The listing builds one solid part. Answer for the finished solid, in the listing's coordinates (mm). Face numbers are marked on the shaded views. A direction names the side the tool comes from. Round coordinates to 2 decimals unless told otherwise and drop trailing zeros. Write each loop counter-clockwise with the first axis right and the second up, starting at its lowest first coordinate (ties: lowest second). Pieces come first, ordered by that corner, then holes.
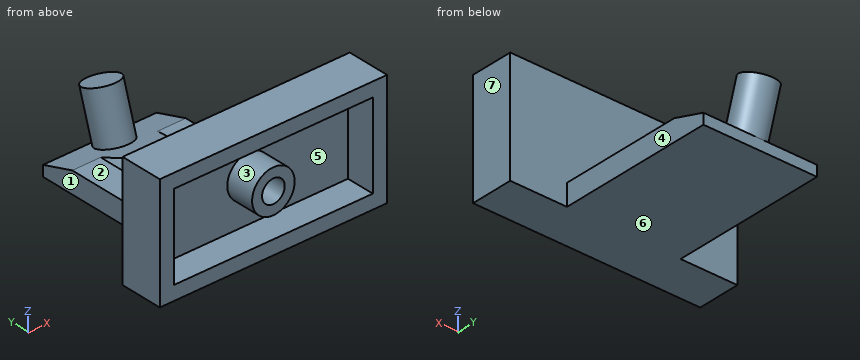
from build123d import *

# Parameters (mm, degrees)
SKETCH1_W           = 16
SKETCH1_H           = 8
BOSS_EXTRUDE1_DEPTH = 3
SHELL1_T            = -1
SKETCH2_R           = 1.5
SKETCH2_R_2         = 0.8
BOSS_EXTRUDE2_DEPTH = 2
BOSS_EXTRUDE3_DEPTH = 11
CUT_EXTRUDE2_DEPTH  = 13
SKETCH6_R           = 1.2
BOSS_EXTRUDE4_DEPTH = 3.5


with BuildPart() as part:
    # Sketch1 → Boss-Extrude1 (new body)
    with BuildSketch(Plane(origin=(0, 0, 0), x_dir=(1, 0, 0), z_dir=(0, 1, 0))):
        Rectangle(SKETCH1_W, SKETCH1_H)
    extrude(amount=BOSS_EXTRUDE1_DEPTH)

    # Shell1
    shell1_openings = [part.faces().sort_by_distance(p)[0] for p in [
        (0, 0, 0),
    ]]
    offset(amount=SHELL1_T, openings=shell1_openings, kind=Kind.INTERSECTION)

    # Sketch2 → Boss-Extrude2 (add)
    with BuildSketch(Plane.XZ.offset(-2)):
        Circle(SKETCH2_R)
        Circle(SKETCH2_R_2, mode=Mode.SUBTRACT)
    extrude(amount=BOSS_EXTRUDE2_DEPTH)

    # Sketch3 → Boss-Extrude3 (add)
    with BuildSketch(Plane(origin=(0, 3, 0), x_dir=(1, 0, 0), z_dir=(0, 1, 0))):
        with BuildLine():
            Line((-4, 4), (4, 4))
            Line((4, 4), (4, 2.5))
            Line((4, 2.5), (2, 2.5))
            ThreePointArc((2, 2.5), (0, 1.5), (-2, 2.5))
            Line((-2, 2.5), (-4, 2.5))
            Line((-4, 2.5), (-4, 4))
        make_face()
    extrude(amount=BOSS_EXTRUDE3_DEPTH)

    # Sketch5 → Cut-Extrude2 (cut, through all)
    with BuildSketch(Plane(origin=(4, 0, 0), x_dir=(0, 0, -1), z_dir=(1, 0, 0))):
        Polygon((3.25, 14), (1.5, 14), (1.5, 8.5), align=None)
    extrude(amount=-CUT_EXTRUDE2_DEPTH, mode=Mode.SUBTRACT)

    # Sketch6 → Boss-Extrude4 (add)
    with BuildSketch(Plane(origin=(0, 0.348030019, 1.09380863), x_dir=(1, 0, 0), z_dir=(0, 0.303203657, 0.95292578))):
        with Locations((0, 13.089580337)):
            Circle(SKETCH6_R)
    extrude(amount=BOSS_EXTRUDE4_DEPTH)


solid = part.part
1. For a pull along X with two mould halves and no side action, classify the marked faces 5, 6 and 7 as released by +X, released by -X, zero draft, split by the parting line, or undercut.
Geometry says:
face 5: undercut
face 6: zero draft
face 7: released by +X
2. A tool of negligible diameter and unlimited length cuts with its end or side. For the marked faces 1, 2, 3 and 4, from which of +Z, -Z, +X, -X, +Y, -Y can it reach the whole face along a straight path? Write none if from no direction.
Geometry says:
face 1: +Z, -Z, -X, +Y
face 2: +Z, -X, +Y
face 3: -Y
face 4: +Z, -Z, +X, +Y
3. Section B-B on y = 9.5 is taken. Determine the outline of the cut face in (x, z).
Geometry says:
outline: (-4, -4) - (4, -4) - (4, -2.5) - (2, -2.5) arc R2.5 ccw to (1.22, -1.82) - (-1.22, -1.82) arc R2.5 ccw to (-2, -2.5) - (-4, -2.5) - close
4. Section D-D on x = 6 is taken. Determine the outline of the cut face in (y, z).
Geometry says:
outline: (0, -4) - (3, -4) - (3, 4) - (0, 4) - (0, 3) - (2, 3) - (2, -3) - (0, -3) - close
5. Straight lines are drawn through the part: line 1 along Z through (x, y) = (0, 1); line 2 along Z through (x, y) = (-1.25, 1.25); line 3 along Y through (x, z) = (-6, -2.5). For each, find the intervals that lie inside material, in ascending order.
Geometry says:
line 1: z = -4 to -3, -1.5 to -0.8, 0.8 to 1.5, 3 to 4
line 2: z = -4 to -3, -0.83 to 0.83, 3 to 4
line 3: y = 2 to 3
6. Given pin 1 (0.8 mm diameter, centred on y = 9.5, z = -3, fed in from -X); pin 2 (1 mm diameter, centred on x = -1, z = -3, fed in from +Y); pin 3 (2 mm diameter, centred on x = 3.5, y = 9, fed in from +Z); pin 4 (2.5 mm diameter, centred on x = 0, z = 0, fed in from +Y), each flat-ended and moving along its own axis, determine where each tip first touches the part or whether it passes through.
Geometry says:
pin 1: stops at x = -4
pin 2: stops at y = 14
pin 3: stops at z = -2.5
pin 4: stops at y = 15.03
7. Section A-A on x = -2.5 is taken. Determine the outline of the cut face in (y, z).
Geometry says:
outline: (0, -4) - (14, -4) - (14, -3.25) - (11.64, -2.5) - (3, -2.5) - (3, 4) - (0, 4) - (0, 3) - (2, 3) - (2, -3) - (0, -3) - close
8. Section C-C on z = 3.75 is taken. Determine the outline of the cut face in (x, y), plus the area to 3 significant figures.
Geometry says:
outline: (-8, 0) - (8, 0) - (8, 3) - (-8, 3) - close
area: 48.0 mm2
